Source: CAD feature listing. Evaluate the final solid. Frame: model axes, mm. Face numbers are marked on the shaded views. A direction names the side the tool comes from. Give positions to 0.01 mm unless a question says otherwise; leave off trailing zeros. Order: outer loops, then holes, each group sorted by start corner. A loop starts at its lowest first (then second) coordinate and runs counter-clockwise, first axis right, second up.
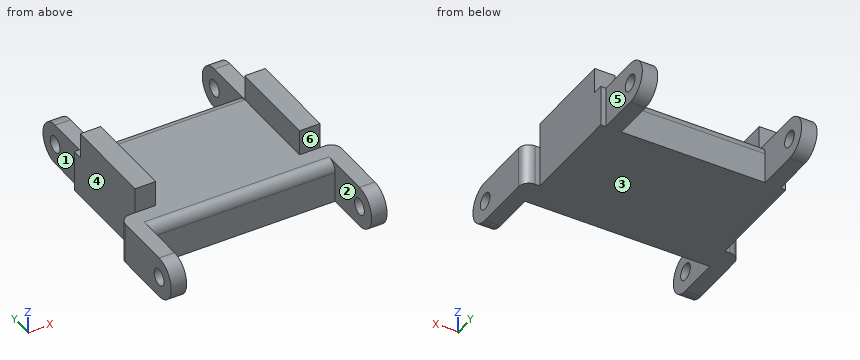
from build123d import *

# Parameters (mm, degrees)
SKETCH_1_W      = 36
SKETCH_1_H      = 25
EXTRUDE_1_DEPTH = 8
EXTRUDE_START   = -1
SKETCH_2_R      = 1.6
EXTRUDE_2_DEPTH = 3
EXTRUDE_START_2 = -32
SKETCH_2_3_R    = 1.6
EXTRUDE_3_DEPTH = 3
SKETCH_4_R      = 1.6
EXTRUDE_4_DEPTH = 3
FILLET_2_R      = 2
EXTRUDE_START_3 = -39
SKETCH_4_3_R    = 1.6
EXTRUDE_5_DEPTH = 3
FILLET_3_R      = 2
FILLET_4_R      = 2
FILLET_5_R      = 2
SKETCH_5_W      = 4
SKETCH_5_H      = 18
EXTRUDE_6_DEPTH = 5


with BuildPart() as part:
    # Эскиз1 → Бобышка-Вытянуть1 (new body)
    with BuildSketch(Plane.XY):
        with Locations((18, 12.5)):
            Rectangle(SKETCH_1_W, SKETCH_1_H)
    extrude(amount=EXTRUDE_1_DEPTH)

    # Эскиз2 → Бобышка-Вытянуть2 (add)
    with BuildSketch(Plane(origin=(36, 0, 0), x_dir=(0, 0, -1), z_dir=(1, 0, 0)).offset(EXTRUDE_START)):
        with BuildLine():
            Line((-8, 25), (0, 25))
            Line((0, 25), (0, 33))
            ThreePointArc((0, 33), (-4, 37), (-8, 33))
            Line((-8, 33), (-8, 25))
        make_face()
        with Locations((-4, 33)):
            Circle(SKETCH_2_R, mode=Mode.SUBTRACT)
    extrude(amount=-EXTRUDE_2_DEPTH)

    # Эскиз2<3> → Бобышка-Вытянуть3 (add)
    with BuildSketch(Plane(origin=(36, 0, 0), x_dir=(0, 0, -1), z_dir=(1, 0, 0)).offset(EXTRUDE_START_2)):
        with BuildLine():
            Line((-8, 25), (0, 25))
            Line((0, 25), (0, 33))
            ThreePointArc((0, 33), (-4, 37), (-8, 33))
            Line((-8, 33), (-8, 25))
        make_face()
        with Locations((-4, 33)):
            Circle(SKETCH_2_3_R, mode=Mode.SUBTRACT)
    extrude(amount=-EXTRUDE_3_DEPTH)

    # Эскиз4 → Бобышка-Вытянуть4 (add)
    with BuildSketch(Plane.ZY):
        with BuildLine():
            Line((8, -8), (8, 5))
            Line((8, 5), (0, 5))
            Line((0, 5), (0, -8))
            ThreePointArc((0, -8), (4, -12), (8, -8))
        make_face()
        with Locations((4, -8)):
            Circle(SKETCH_4_R, mode=Mode.SUBTRACT)
    extrude(amount=EXTRUDE_4_DEPTH)

    # Скругление2
    fillet_2_edges = [part.edges().sort_by_distance(p)[0] for p in [
        (-3, 5, 4),
    ]]
    fillet(fillet_2_edges, radius=FILLET_2_R)

    # Эскиз4<3> → Бобышка-Вытянуть5 (add)
    with BuildSketch(Plane.ZY.offset(EXTRUDE_START_3)):
        with BuildLine():
            Line((8, -8), (8, 5))
            Line((8, 5), (0, 5))
            Line((0, 5), (0, -8))
            ThreePointArc((0, -8), (4, -12), (8, -8))
        make_face()
        with Locations((4, -8)):
            Circle(SKETCH_4_3_R, mode=Mode.SUBTRACT)
    extrude(amount=EXTRUDE_5_DEPTH)

    # Скругление3
    fillet_3_edges = [part.edges().sort_by_distance(p)[0] for p in [
        (39, 5, 4),
    ]]
    fillet(fillet_3_edges, radius=FILLET_3_R)

    # Скругление4
    fillet_4_edges = [part.edges().sort_by_distance(p)[0] for p in [
        (18, 0, 8),
    ]]
    fillet(fillet_4_edges, radius=FILLET_4_R)

    # Скругление5
    fillet_5_edges = [part.edges().sort_by_distance(p)[0] for p in [
        (18, 25, 8),
    ]]
    fillet(fillet_5_edges, radius=FILLET_5_R)

    # Эскиз5 → Бобышка-Вытянуть6 (add)
    with BuildSketch(Plane.XY.offset(8)):
        with Locations((2, 14)):
            Rectangle(SKETCH_5_W, SKETCH_5_H)
        with Locations((34, 14)):
            Rectangle(SKETCH_5_W, SKETCH_5_H)
    extrude(amount=EXTRUDE_6_DEPTH)


solid = part.part
1) Section query A-A on z = 12. Output: boundary loops of the cut face in (x, y).
Checks:
outline: (0, 5) - (4, 5) - (4, 23) - (0, 23) - close; (32, 5) - (36, 5) - (36, 23) - (32, 23) - close
2) Section query B-B on x = 16. Output: boundary loops of the cut face in (y, z).
Checks:
outline: (0, 0) - (25, 0) - (25, 6) arc R2 ccw to (23, 8) - (2, 8) arc R2 ccw to (0, 6) - close
3) Ray query, L1, parallel to X at y = 16.5, z = 10.75; L2, parallel to X at y = 29.5, z = 2.25; L3, parallel to Y at x = 2.45, z = 4. Return the intervals inside material, ascending.
Checks:
L1: x = 0 to 4, 32 to 36
L2: x = 1 to 4, 32 to 35
L3: y = 0 to 31.4, 34.6 to 37
4) Section query C-C on z = 4. State how many separate pieces and enclosed holes the cut face has, and give its area (3 significant figures).
Checks:
separate pieces: 5
enclosed holes: 0
area: 1,030 mm2
5) Pull-direction query (X, two-part tool) for the marked faces 1, 2 and 3; classes: +X half, -X half, draft (parallel to the pull), parting line (faces both ways), or undercut.
Checks:
face 1: -X half
face 2: undercut
face 3: draft
6) Section query D-D on z = 1.25. Output: boundary loops of the cut face in (x, y).
Checks:
outline: (-3, -10.9) - (0, -10.9) - (0, 0) - (36, 0) - (36, -10.9) - (39, -10.9) - (39, 3) arc R2 ccw to (37, 5) - (36, 5) - (36, 25) - (35, 25) - (35, 35.9) - (32, 35.9) - (32, 25) - (4, 25) - (4, 35.9) - (1, 35.9) - (1, 25) - (0, 25) - (0, 5) - (-1, 5) arc R2 ccw to (-3, 3) - close
7) Reachability of the marked faces 4, 5 and 6 from +Z, -Z, +X, -X, +Y, -Y: full face, straight path, thin tool, end or side. Return the list, or none.
Checks:
face 4: +Z, -Z, -X, +Y
face 5: +Z, -Z, +X, +Y
face 6: +Z, +X, -X, -Y
8) First-contact query: pin 1 Ø2.5 at (y, z) = (33, 4) entering from +X; pin 2 Ø1.2 at (x, y) = (34, 28) entering from +Z; pin 3 Ø2 at (x, z) = (2.5, 11) entering from -Y; pin 4 Ø1.5 at (x, z) = (31.5, 7) entering from +Y. Flat tips, straight axial feed; report the tip coordinate or a pass-through.
Checks:
pin 1: passes through
pin 2: stops at z = 8
pin 3: stops at y = 5
pin 4: stops at y = 36.17
